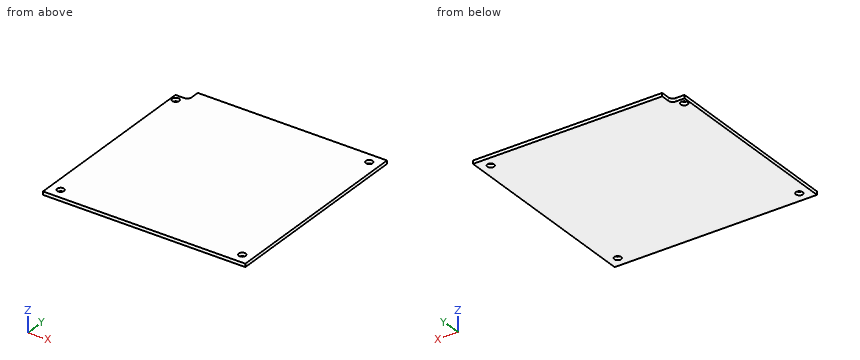
```python
from build123d import *

# Parameters (mm, degrees)
SKETCH1_W                  = 92.5
SKETCH1_H                  = 92.5
BOSS_EXTRUDE1_DEPTH        = 1.5
F_3_1_3_1_DIAMETER_HOLE1_D = 3.1
CUT_EXTRUDE1_DEPTH         = 10


with BuildPart() as part:
    # Sketch1 → Boss-Extrude1 (new body)
    with BuildSketch(Plane.XY):
        Rectangle(SKETCH1_W, SKETCH1_H)
    extrude(amount=BOSS_EXTRUDE1_DEPTH)

    # Ø3.1 (3.1) Diameter Hole1 (through all)
    with Locations(Plane.XY.offset(1.5)):
        with Locations((-44.05, 37.328004442), (41.5, 41.5), (41.5, -41.5), (-41.5, -41.5)):
            Hole(F_3_1_3_1_DIAMETER_HOLE1_D / 2)

    # Sketch6 → Cut-Extrude1 (cut)
    with BuildSketch(Plane(origin=(0, 0, 0), x_dir=(-1, 0, 0), z_dir=(0, 0, -1))):
        with BuildLine():
            Line((46.25, 46.25), (40.25, 46.25))
            Line((40.25, 46.25), (40.25, 42.25))
            ThreePointArc((40.25, 42.25), (40.835786438, 40.835786438), (42.25, 40.25))
            Line((42.25, 40.25), (46.25, 40.25))
            Line((46.25, 40.25), (46.25, 46.25))
        make_face()
    extrude(amount=-CUT_EXTRUDE1_DEPTH, mode=Mode.SUBTRACT)


solid = part.part
```
CAD build for the part. Positions are in the model's coordinates, mm. Round coordinates to 2 decimals unless told otherwise and drop trailing zeros. Write each loop counter-clockwise with the first axis right and the second up, starting at its lowest first coordinate (ties: lowest second). Pieces come first, ordered by that corner, then holes. Notation, with made-up numbers: M -31,4 L 23,4 A17 cw 23,32 Z; hole C 47.25,60 d5. An arc over 180 degrees is marked long. One line per question, with ' | ' between items.
1. Probe L1, parallel to Y at x = 41.5, z = 1.1; L2, parallel to Y at x = -44.05, z = 0.55; L3, parallel to X at y = 36, z = 0.2. List the from-to ranges inside material, lowest first. Write a range as from..to.
Working result:
L1: -46.25..-43.05, -39.95..39.95, 43.05..46.25 | L2: -46.25..35.78, 38.88..40.25 | L3: -46.25..-44.85, -43.25..46.25
2. Pin check, flat tip, straight feed: pin 1 Ø0.8 at (y, z) = (44.5, 0.5) entering from -X. Stop position of the tip, or through.
Working result:
pin 1: x = -40.25
3. Cut at A-A on y = -41.5. Write the cut outline in (x, z), and give its area (3 significant figures).
Working result:
outline: M -46.25,0 L -43.05,0 L -43.05,1.5 L -46.25,1.5 Z; M -39.95,0 L 39.95,0 L 39.95,1.5 L -39.95,1.5 Z; M 43.05,0 L 46.25,0 L 46.25,1.5 L 43.05,1.5 Z | area: 129 mm2
